from build123d import *

# Parameters (mm, degrees)
BOSS_EXTRUDE1_DEPTH = 22.5
FILLET1_R           = 12
CUT_EXTRUDE1_START  = 5.5
SCREW_MOUNT_R       = 2.8
SCREW_MOUNT_R_2     = 1.625
CUT_EXTRUDE1_DEPTH  = 2
CUT_EXTRUDE2_START  = 5
SCREW_MOUNT_3_R     = 1.625
CUT_EXTRUDE2_DEPTH  = 76.508864857
FILLET3_R           = 2
FILLET4_R           = 2


with BuildPart() as part:
    # Base → Boss-Extrude1 (new body)
    with BuildSketch(Plane.XY):
        Polygon((-27.725, 0), (-10.225, 0), (-6.25, 7), (6.25, 7), (10.225, 0), (27.725, 0), (47, 10), (47, 37.5), (18.975, 47.5), (-18.975, 47.5), (-47, 37.5), (-47, 10), align=None)
        with BuildLine():
            Line((-28.670726654, 6.123500417), (-36.605187851, 10.2399524))
            ThreePointArc((-36.605187851, 10.2399524), (-40.545521591, 13.922796166), (-42, 19.116451983))
            Line((-42, 19.116451983), (-42, 26.926039841))
            ThreePointArc((-42, 26.926039841), (-40.17334162, 32.687679084), (-35.360702646, 36.344409006))
            Line((-35.360702646, 36.344409006), (-19.7396793, 41.918369165))
            ThreePointArc((-19.7396793, 41.918369165), (-18.084307759, 42.353519464), (-16.378976654, 42.5))
            Line((-16.378976654, 42.5), (16.378976654, 42.5))
            ThreePointArc((16.378976654, 42.5), (18.084307759, 42.353519464), (19.7396793, 41.918369165))
            Line((19.7396793, 41.918369165), (35.360702646, 36.344409006))
            ThreePointArc((35.360702646, 36.344409006), (40.17334162, 32.687679084), (42, 26.926039841))
            Line((42, 26.926039841), (42, 19.116451983))
            ThreePointArc((42, 19.116451983), (40.545521591, 13.922796166), (36.605187851, 10.2399524))
            Line((36.605187851, 10.2399524), (28.670726654, 6.123500417))
            ThreePointArc((28.670726654, 6.123500417), (26.435665821, 5.284934487), (24.065538803, 5))
            Line((24.065538803, 5), (13.1356311, 5))
            Line((13.1356311, 5), (12.035146877, 6.937959637))
            ThreePointArc((12.035146877, 6.937959637), (8.370293449, 10.642325971), (3.3393689, 12))
            Line((3.3393689, 12), (-3.3393689, 12))
            ThreePointArc((-3.3393689, 12), (-8.370293449, 10.642325971), (-12.035146877, 6.937959637))
            Line((-12.035146877, 6.937959637), (-13.1356311, 5))
            Line((-13.1356311, 5), (-24.065538803, 5))
            ThreePointArc((-24.065538803, 5), (-26.435665821, 5.284934487), (-28.670726654, 6.123500417))
        make_face(mode=Mode.SUBTRACT)
    extrude(amount=BOSS_EXTRUDE1_DEPTH)

    # Fillet1
    fillet1_edges = [part.edges().sort_by_distance(p)[0] for p in [
        (13.1356311, 5, 11.25),
        (-13.1356311, 5, 11.25),
    ]]
    fillet(fillet1_edges, radius=FILLET1_R)

    # Screw_Mount → Cut-Extrude1 (cut)
    with BuildSketch(Plane(origin=(0, 0, 0), x_dir=(1, 0, 0), z_dir=(0, 1, 0)).offset(CUT_EXTRUDE1_START)):
        with Locations(Location((-18.975, -11.25, 0), (0, 0, 270))):
            Circle(SCREW_MOUNT_R)
        with Locations((-18.975, -11.25)):
            Circle(SCREW_MOUNT_R_2, mode=Mode.SUBTRACT)
        with Locations((-18.975, -11.25)):
            Circle(SCREW_MOUNT_R_2)
        with Locations(Location((18.975, -11.25, 0), (0, 0, 270))):
            Circle(SCREW_MOUNT_R)
        with Locations((18.975, -11.25)):
            Circle(SCREW_MOUNT_R_2, mode=Mode.SUBTRACT)
        with Locations((18.975, -11.25)):
            Circle(SCREW_MOUNT_R_2)
    extrude(amount=-CUT_EXTRUDE1_DEPTH, mode=Mode.SUBTRACT)

    # Screw_Mount<3> → Cut-Extrude2 (cut, through all)
    with BuildSketch(Plane(origin=(0, 0, 0), x_dir=(1, 0, 0), z_dir=(0, 1, 0)).offset(CUT_EXTRUDE2_START)):
        with Locations(Location((-18.975, -11.25, 0), (0, 0, 270))):
            Circle(SCREW_MOUNT_3_R)
        with Locations(Location((18.975, -11.25, 0), (0, 0, 270))):
            Circle(SCREW_MOUNT_3_R)
    extrude(amount=-CUT_EXTRUDE2_DEPTH, mode=Mode.SUBTRACT)

    # Fillet3
    fillet3_edges = [part.edges().sort_by_distance(p)[0] for p in [
        (-47, 10, 11.25),
        (-47, 37.5, 11.25),
        (-18.975, 47.5, 11.25),
        (47, 37.5, 11.25),
        (47, 10, 11.25),
        (27.725, 0, 11.25),
        (10.225, 0, 11.25),
        (6.25, 7, 11.25),
        (-6.25, 7, 11.25),
        (-10.225, 0, 11.25),
        (-27.725, 0, 11.25),
    ]]
    fillet(fillet3_edges, radius=FILLET3_R)

    # Fillet4
    fillet4_edges = [part.edges().sort_by_distance(p)[0] for p in [
        (21.749192321, 5, 22.5),
        (-7.327989076, 11.170109546, 22.5),
        (14.646501628, 5.995868544, 22.5),
        (-14.646501628, 5.995868544, 22.5),
        (26.435665821, 5.284934487, 22.5),
        (32.637957253, 8.181726408, 22.5),
        (40.545521591, 13.922796166, 22.5),
        (42, 23.021245912, 22.5),
        (40.17334162, 32.687679084, 22.5),
        (27.550190973, 39.131389085, 22.5),
        (18.084307759, 42.353519464, 22.5),
        (0, 42.5, 22.5),
        (-18.084307759, 42.353519464, 22.5),
        (-27.550190973, 39.131389085, 22.5),
        (-40.17334162, 32.687679084, 22.5),
        (-42, 23.021245912, 22.5),
        (-40.545521591, 13.922796166, 22.5),
        (-32.637957253, 8.181726408, 22.5),
        (-26.435665821, 5.284934487, 22.5),
        (-21.749192321, 5, 22.5),
        (0, 12, 22.5),
        (7.327989076, 11.170109546, 22.5),
    ]]
    fillet(fillet4_edges, radius=FILLET4_R)


solid = part.part
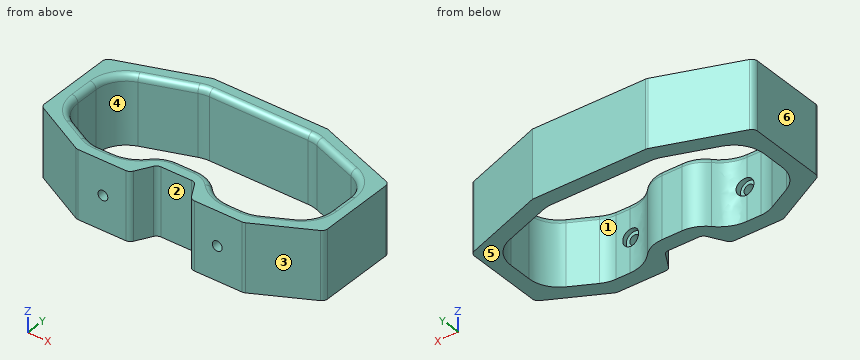
The model under review builds one solid part; all positions refer to its coordinate system, in mm. Face numbers are marked on the shaded views. A direction names the side the tool comes from. Coordinates: 2 decimals unless noted, no trailing zeros. Write each loop counter-clockwise with the first axis right and the second up, starting at its lowest first coordinate (ties: lowest second). Pieces come first, ordered by that corner, then holes. Notation, with made-up numbers: (77.25, 82) - (124.25, 82) arc R29 cw to (124.25, 120) - close; hole circle Ø1 at (80.5, 27.5). An arc over 180 degrees is marked (long way). Answer as a JSON object with one key per item and string values. Group by question number.
1. To check wall thickness, follow probe 1 along X at (y, z) = (20.5, 7); probe 2 along X at (y, z) = (4.35, 11.25) (3 decimals); probe 3 along X at (y, z) = (2.1, 11.25). State the ranges of each line that lie inside material, in increasing order.
2. Machinability: for the marked faces 1, 2 and 3, which of the approach directions +Z, -Z, +X, -X, +Y, -Y give a long, thin tool a straight path to every point of the face, cutting with its end or side? Answer none if there is none.
3. Mouldability with a two-part tool opening along X and no side actions: class the marked faces 4, 5 and 6 as pulls with the +X half, pulls with the -X half, needs draft (parallel to the pull), parting line crosses it, or undercut.
4. Clearance check with flat-ended pins moving along their axes: pin 1 Ø8 at (x, z) = (0, 14.5) entering from -Y; pin 2 Ø3 at (x, z) = (-18.975, 11.25) entering from -Y; pin 3 Ø3.5 at (x, z) = (22, 11.5) entering from +Y. State where each tip first meets the part, or that it passes through.
5. Add section A-A (y = 20). Give the boundary of the cut face in (x, z), plus the area to 3 significant figures.
6. Add section B-B (x = 1). Give the boundary of the cut face in (y, z), plus the area to 3 significant figures.
Findings:
{
 "1": {"probe 1": "-47 to -42, 42 to 47", "probe 2": "-36.11 to -21.775, -16.175 to -7.755, 7.755 to 16.175, 21.775 to 36.11", "probe 3": "-31.77 to -20.6, -17.35 to -9.03, 9.03 to 17.35, 20.6 to 31.77"},
 "2": {"face 1": "+Z, -Z", "face 2": "+Z, -Z, -Y", "face 3": "+Z, -Z, +X, -Y"},
 "3": {"face 4": "undercut", "face 5": "needs draft", "face 6": "pulls with the -X half"},
 "4": {"pin 1": "y = 7", "pin 2": "y = 41.66", "pin 3": "y = 47.05"},
 "5": {"outline": "(-47, 0) - (-42, 0) - (-42, 20.5) arc R2 ccw to (-44, 22.5) - (-47, 22.5) - close; (42, 0) - (47, 0) - (47, 22.5) - (44, 22.5) arc R2 ccw to (42, 20.5) - close", "area": "223 mm²"},
 "6": {"outline": "(7, 0) - (12, 0) - (12, 20.5) arc R2 ccw to (10, 22.5) - (7, 22.5) - close; (42.5, 0) - (47.5, 0) - (47.5, 22.5) - (44.5, 22.5) arc R2 ccw to (42.5, 20.5) - close", "area": "223 mm²"}
}
